Check sheet for the modelled part. Datum: model origin and axes. Units: mm. Face numbers are marked on the shaded views. A direction names the side the tool comes from. Round coordinates to 2 decimals unless told otherwise and drop trailing zeros. Loops run counter-clockwise (first coordinate to the right, second up) from the corner with the lowest first, then second, coordinate; pieces in that order, holes last. Notation, with made-up numbers: (-39.5, 49.25) - (13.5, 49.25) arc R23 cw to (13.5, 64.25) - close; hole circle Ø1 at (10.5, 45.25). An arc over 180 degrees is marked (long way). Answer in a Markdown table with one row per item. Add a question column.
(1) Gauge pin test, flat ends, axial feed: pin 1 (2 mm diameter, centred on x = -6.5, z = 28.5, fed in from +Y); pin 2 (1 mm diameter, centred on x = -12.5, y = -153.5, fed in from +Z); pin 3 (5.5 mm diameter, centred on y = -128, z = 39.5, fed in from +X). Record the tip position at first contact, or that the pin passes through.
(2) Access from +Z, -Z, +X, -X, +Y, -Y to the whole of each face (thin tool, end or side, straight path). Record for the marked faces 4, 5, 6 and 7.
(3) Mould release check, pull along X, two halves, no side actions. Record for the marked faces 1, 2 and 3: +X half, -X half, draft (parallel to the pull), parting line (faces both ways), or undercut.
(4) Cross-section at B-B on y = -230. Enter the section's corners in (x, z).
(5) Thickness scan on line 1 along X through (y, z) = (-31, 7); line 2 along Y through (x, z) = (0, 15.5); line 3 along Y through (x, z) = (-4, 35.5). Record the ranges inside material, lowest first.
(6) Cross-section at C-C on z = 42. Enter the section's corners in (x, y), then the cut area to 3 significant figures.
(7) Cross-section at A-A on x = 0. Enter the section's corners in (y, z), then the cut area to 3 significant figures.
from build123d import *

# Parameters (mm, degrees)
SKETCH2_W           = 20
SKETCH2_H           = 220
BOSS_EXTRUDE1_DEPTH = 20
SKETCH3_W           = 60
SKETCH3_H           = 20
BOSS_EXTRUDE2_DEPTH = 30
SKETCH4_W           = 70
SKETCH4_H           = 30
SKETCH4_W_2         = 60
SKETCH4_H_2         = 20
BOSS_EXTRUDE3_DEPTH = 10
FILLET1_R           = 1
FILLET2_R           = 1
FILLET3_R           = 1


with BuildPart() as part:
    # Sketch2 → Boss-Extrude1 (new body)
    with BuildSketch(Plane.XY):
        with BuildLine():
            Line((30, 0), (30, -100))
            Line((30, -100), (40, -100))
            Line((40, -100), (40, -160))
            Line((40, -160), (30, -160))
            Line((30, -160), (30, -260))
            ThreePointArc((30, -260), (0, -290), (-30, -260))
            Line((-30, -260), (-30, -160))
            Line((-30, -160), (-40, -160))
            Line((-40, -160), (-40, -100))
            Line((-40, -100), (-30, -100))
            Line((-30, -100), (-30, 0))
            ThreePointArc((-30, 0), (0, 30), (30, 0))
        make_face()
        with Locations((0, -130)):
            Rectangle(SKETCH2_W, SKETCH2_H, mode=Mode.SUBTRACT)
    extrude(amount=BOSS_EXTRUDE1_DEPTH)

    # Sketch3 → Boss-Extrude2 (add)
    with BuildSketch(Plane.XY.offset(20)):
        with Locations((0, -130)):
            Rectangle(SKETCH3_W, SKETCH3_H)
    extrude(amount=BOSS_EXTRUDE2_DEPTH)

    # Sketch4 → Boss-Extrude3 (add)
    with BuildSketch(Plane.XY.offset(20)):
        with Locations((0, -130)):
            Rectangle(SKETCH4_W, SKETCH4_H)
        with Locations((0, -130)):
            Rectangle(SKETCH4_W_2, SKETCH4_H_2, mode=Mode.SUBTRACT)
    extrude(amount=BOSS_EXTRUDE3_DEPTH)

    # Fillet1
    fillet1_edges = [part.edges().sort_by_distance(p)[0] for p in [
        (30, -130, 50),
        (0, -120, 50),
        (-30, -130, 50),
        (0, -140, 50),
        (35, -130, 30),
        (0, -115, 30),
        (-35, -130, 30),
        (0, -145, 30),
        (0, -140, 30),
        (30, -130, 30),
        (0, -120, 30),
        (-30, -130, 30),
    ]]
    fillet(fillet1_edges, radius=FILLET1_R)

    # Fillet2
    fillet2_edges = [part.edges().sort_by_distance(p)[0] for p in [
        (30, -50, 0),
        (40, -130, 0),
        (30, -210, 0),
        (0, -290, 0),
        (-30, -210, 0),
        (-40, -130, 0),
        (-30, -50, 0),
        (0, 30, 0),
        (-40, -130, 20),
        (-30, -210, 20),
        (0, -290, 20),
        (30, -210, 20),
        (40, -130, 20),
        (30, -50, 20),
        (0, 30, 20),
        (-30, -50, 20),
    ]]
    fillet(fillet2_edges, radius=FILLET2_R)

    # Fillet3
    fillet3_edges = [part.edges().sort_by_distance(p)[0] for p in [
        (-34, -160, 0),
        (-39.707106781, -160, 0.292893219),
        (-40, -160, 10),
        (-39.707106781, -160, 19.707106781),
        (34, -160, 0),
        (39.707106781, -160, 0.292893219),
        (40, -160, 10),
        (39.707106781, -160, 19.707106781),
        (34, -100, 0),
        (39.707106781, -100, 0.292893219),
        (40, -100, 10),
        (39.707106781, -100, 19.707106781),
        (-34, -100, 0),
        (-39.707106781, -100, 0.292893219),
        (-40, -100, 10),
        (-39.707106781, -100, 19.707106781),
        (-34, -160, 20),
        (34, -160, 20),
        (34, -100, 20),
        (-34, -100, 20),
    ]]
    fillet(fillet3_edges, radius=FILLET3_R)


solid = part.part
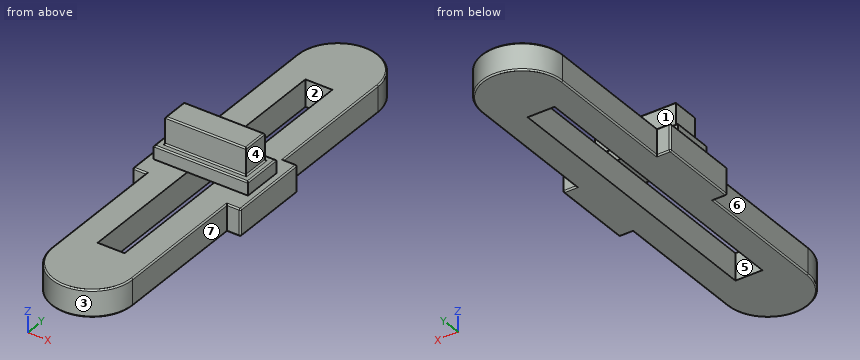
Answers:
| question | item | result |
|---|---|---|
| 1 | pin 1 | stops at y = -115 |
| 1 | pin 2 | stops at z = 20 |
| 1 | pin 3 | stops at x = 30 |
| 2 | face 4 | +Z, +X, +Y, -Y |
| 2 | face 5 | +Z, -Z |
| 2 | face 6 | +Z, -Z, -X, -Y |
| 2 | face 7 | +Z, -Z, +X, -Y |
| 3 | face 1 | draft |
| 3 | face 2 | undercut |
| 3 | face 3 | parting line |
| 4 | outline | (-30, 1) arc R1 ccw to (-29, 0) - (-10, 0) - (-10, 20) - (-29, 20) arc R1 ccw to (-30, 19) - close; (10, 0) - (29, 0) arc R1 ccw to (30, 1) - (30, 19) arc R1 ccw to (29, 20) - (10, 20) - close |
| 5 | line 1 | x = -30 to -10, 10 to 30 |
| 5 | line 2 | y = -290 to -240, -20 to 30 |
| 5 | line 3 | y = -140 to -120 |
| 6 | outline | (-30, -140) - (30, -140) - (30, -120) - (-30, -120) - close |
| 6 | area | 1,200 mm^2 |
| 7 | outline | (-290, 1) arc R1 ccw to (-289, 0) - (-240, 0) - (-240, 20) - (-289, 20) arc R1 ccw to (-290, 19) - close; (-145, 20) - (-115, 20) - (-115, 29) arc R1 ccw to (-116, 30) - (-119, 30) arc R1 cw to (-120, 31) - (-120, 49) arc R1 ccw to (-121, 50) - (-139, 50) arc R1 ccw to (-140, 49) - (-140, 31) arc R1 cw to (-141, 30) - (-144, 30) arc R1 ccw to (-145, 29) - close; (-20, 0) - (29, 0) arc R1 ccw to (30, 1) - (30, 19) arc R1 ccw to (29, 20) - (-20, 20) - close |
| 7 | area | 2,700 mm^2 |
